Autodesk Inventor part; units mm, degrees
ref_plane "YZ Plane" through (0, 0, 0) normal (1, 0, 0) x (0, 1, 0)
ref_plane "XZ Plane" through (0, 0, 0) normal (0, 1, 0) x (-1, 0, 0)
ref_plane "XY Plane" through (0, 0, 0) normal (0, 0, 1) x (1, 0, 0)
sketch "Skizze1" plane through (0, 0, 0) normal (0, 0, 1) x (1, 0, 0)
  line L0 (-75.636, -5) -> (-69.636, -5)
  line L1 (-69.636, -5) -> (-69.636, 5)
  line L2 (-69.636, 5) -> (-75.636, 5)
  line L3 (-75.636, 5) -> (-75.636, -5)
  line L4 (-72.636, -5) -> (-72.636, 0) construction
  line L5 (-72.636, 0) -> (-72.636, 5) construction
  line L6 (0, 0) -> (-72.636, 0) construction
  line L7 (-65.022, 4) -> (-65.022, -4) construction
  line L8 (-65.022, 4) -> (-65.022, -4) construction
  line L9 (-65.022, 4) -> (-65.022, -4) construction
  point P0 (-63.636, 3)
  dimension "d0" = 6
  dimension "d1" = 10
  dimension "d2" = 6
extrude "Extrusion1" add sketch "Skizze1" along normal blind 5.5
sketch "Skizze2" plane through (-69.636, -5, 0) normal (1, 0, 0) x (0, 0, -1)
  line L0 (0, 2.65) -> (-4.7, 2.65)
  line L1 (-4.7, 2.65) -> (-4.7, 7.35)
  line L2 (-4.7, 7.35) -> (0, 7.35)
  line L3 (0, 7.35) -> (0, 2.65)
  line L4 (0, 5) -> (-4.7, 5)
  line L5 (0, 0) -> (0, 10)
  point P0 (0, 5)
  dimension "d5" = 4.7
  dimension "d6" = 4.7
extrude "Extrusion2" cut sketch "Skizze2" against normal blind 2
sketch "Skizze3" plane through (0, 0, 5.5) normal (0, 0, 1) x (1, 0, 0)
  line L0 (-75.636, 5) -> (-75.636, -5)
  line L1 (-73.886, -3.25) -> (-75.636, -3.25) construction
  line L2 (-73.886, 3.25) -> (-75.636, 3.25) construction
  line L3 (-73.886, -3.25) -> (-73.886, -5) construction
  line L4 (-73.886, 3.25) -> (-73.886, 5) construction
  line L5 (-75.636, -5) -> (-69.636, -5) construction
  line L6 (-69.636, 5) -> (-75.636, 5) construction
  point P0 (0, 0)
  dimension "d9" = 1.75
hole "Bohrung1" at (-73.886, 3.25, 5.5) at (-73.886, -3.25, 5.5) direction (0, 0, -1) diameter 2.4 end through all countersink diameter 5 countersink angle 90
properties part number "Federhalter" material "PC/ABS-Kunststoff, 3DDruck, PLA"
Geometry check sheet. Reference: the model listing, model coordinates, mm. A direction names the side the tool comes from. Round coordinates to 2 decimals unless told otherwise and drop trailing zeros. Write each loop counter-clockwise with the first axis right and the second up, starting at its lowest first coordinate (ties: lowest second). Pieces come first, ordered by that corner, then holes. Notation, with made-up numbers: (-17.5, 82.25) -> (38.5, 82.25) arc R17 ccw to (38.5, 107.25) -> close; hole circle Ø4 at (-12.75, 34.25). An arc over 180 degrees is marked (long way). One line per item, written item: value. Start each with the question number.
(1) Scan lines: line 1 (X direction, y = -3.25, z = 1.35); line 2 (Y direction, x = -73, z = 4.05); line 3 (Z direction, x = -70.75, y = -2). Record each from-to range of solid material in increasing order. Write a range as [from, to].
(2) Cross-section at D-D, the plane y = 0. Record the cut outline in (x, z), and give its area (3 significant figures).
(3) Cross-section at A-A, the plane y = 3.25. Record the cut outline in (x, z).
(4) Draft check along X on faces 1 (the flat face through (-71, 2.35, 2)), 2 (the flat face through (-71.636, 0, 2)), 3 (the conical face through (-72.922, -2.199, 4.426)), 4 (the cylindrical face through (-72.715, 3.51, 2.071)). Enter one of: +X half, -X half, draft (parallel to the pull), parting line (faces both ways), or undercut.
(5) Cross-section at B-B, the plane z = 0.5. Record the cut outline in (x, y).
(6) Go/stop test with a flat-tipped pin: pin 1 Ø0.6 at (x, y) = (-70.5, -0.5) entering from -Z. Record where the tip stops, or that it passes through.
(7) Access from +Z, -Z, +X, -X, +Y, -Y to the whole of each face (thin tool, end or side, straight path). Record for faces 5 (the flat face through (-71, -2.35, 2)), 6 (the flat face through (-73, -5, 3)).
(8) Cross-section at C-C, the plane x = -70.75. Record the cut outline in (y, z), and give its area (3 significant figures).
Answer:
1. line 1: [-75.64, -75.09], [-72.69, -69.64]
1. line 2: [-5, -4.06], [-2.44, 2.44], [4.06, 5]
1. line 3: [4.7, 5.5]
2. outline: (-75.64, 0) -> (-71.64, 0) -> (-71.64, 4.7) -> (-69.64, 4.7) -> (-69.64, 5.5) -> (-75.64, 5.5) -> close
2. area: 23.6 mm²
3. outline: (-75.64, 0) -> (-75.09, 0) -> (-75.09, 4.2) -> (-75.64, 4.75) -> close; (-72.69, 0) -> (-69.64, 0) -> (-69.64, 5.5) -> (-71.39, 5.5) -> (-72.69, 4.2) -> close
4. face 1: draft
4. face 2: +X half
4. face 3: undercut
4. face 4: undercut
5. outline: (-75.64, -5) -> (-69.64, -5) -> (-69.64, -2.35) -> (-71.64, -2.35) -> (-71.64, 2.35) -> (-69.64, 2.35) -> (-69.64, 5) -> (-75.64, 5) -> close; hole circle Ø2.4 at (-73.89, -3.25); hole circle Ø2.4 at (-73.89, 3.25)
6. pin 1: z = 4.7
7. face 5: -Z, +X
7. face 6: +Z, -Z, +X, -X, -Y
8. outline: (-5, 0) -> (-2.35, 0) -> (-2.35, 4.7) -> (2.35, 4.7) -> (2.35, 0) -> (5, 0) -> (5, 5.5) -> (-5, 5.5) -> close
8. area: 32.9 mm²
